The listing builds one solid part. Answer for the finished solid, in the listing's coordinates (mm). A direction names the side the tool comes from. Coordinates: 2 decimals unless noted, no trailing zeros. Order: outer loops, then holes, each group sorted by start corner. A loop starts at its lowest first (then second) coordinate and runs counter-clockwise, first axis right, second up.
```python
from build123d import *

# Parameters (mm, degrees)
F1_DEPTH = 12.7
F2_F1_R  = 5.08
F2_F2_R  = 5.08


with BuildPart() as f1:
    # F0 (on Front) → F1 (new body, symmetric)
    with BuildSketch(Plane.XZ):
        Polygon((152.4, 0), (0, 0), (0, -127), (101.6, -127), (101.6, -78.0620644748), (76.2, -78.0620644748), (76.2, -103.637776798), (50.8, -103.637776798), (50.8, -78.0620644748), (25.4, -78.0620644748), (25.4, -38.1), (127, -38.1), (127, -127), (152.4, -127), align=None)
    extrude(amount=F1_DEPTH, both=True)

    # F2: fillet of radius 5.08 on 40 edges, made by hand

    # F2_f1
    f2_f1_edges = [f1.edges().sort_by_distance(p)[0] for p in [
        (25.4, 0, -78.0620644748),
        (25.4, 0, -38.1),
        (127, 0, -38.1),
        (76.2, 0, -103.637776798),
        (50.8, 0, -103.637776798),
    ]]
    fillet(f2_f1_edges, radius=F2_F1_R)

    # F2_f2
    f2_f2_edges = [f1.edges().sort_by_distance(p)[0] for p in [
        (76.2, -12.7, 0),
        (76.2, 12.7, 0),
        (152.4, 0, 0),
        (0, 0, 0),
        (139.7, -12.7, -127),
        (152.4, 0, -127),
        (127, 0, -127),
        (139.7, 12.7, -127),
        (101.6, 0, -127),
        (50.8, -12.7, -127),
        (101.6, -12.7, -102.5310322374),
        (101.6, 12.7, -102.5310322374),
        (101.6, 0, -78.0620644748),
        (50.8, 12.7, -127),
        (0, 0, -127),
        (63.5, -12.7, -103.637776798),
        (76.2, -12.7, -88.3099206364),
        (50.8, -12.7, -88.3099206364),
        (50.8, 0, -78.0620644748),
        (50.8, 12.7, -88.3099206364),
        (63.5, 12.7, -103.637776798),
        (76.2, 0, -78.0620644748),
        (88.9, 12.7, -78.0620644748),
        (127, -12.7, -85.09),
        (127, 12.7, -85.09),
        (76.2, -12.7, -38.1),
        (25.4, -12.7, -58.0810322374),
        (40.64, -12.7, -78.0620644748),
        (0, -12.7, -63.5),
        (88.9, -12.7, -78.0620644748),
        (40.64, 12.7, -78.0620644748),
        (0, 12.7, -63.5),
        (25.4, 12.7, -58.0810322374),
        (152.4, -12.7, -63.5),
        (152.4, 12.7, -63.5),
        (26.8878975516, 12.7, -76.5741669232),
        (26.8878975516, 12.7, -39.5878975516),
        (26.8878975516, -12.7, -76.5741669232),
        (26.8878975516, -12.7, -39.5878975516),
        (125.5121024484, -12.7, -39.5878975516),
        (125.5121024484, 12.7, -39.5878975516),
        (74.7121024484, 12.7, -102.1498792464),
        (52.2878975516, 12.7, -102.1498792464),
        (52.2878975516, -12.7, -102.1498792464),
        (74.7121024484, -12.7, -102.1498792464),
    ]]
    fillet(f2_f2_edges, radius=F2_F2_R)


solid = f1.part
```
1) A cutting plane is placed at A-A, the plane z = -54. Write down the section's boundary in (x, y), plus the area to 3 significant figures.
2) A cutting plane is placed at C-C, the plane z = -91. Write down the section's boundary in (x, y).
3) A cutting plane is placed at D-D, the plane y = -0.5. Write down the section's boundary in (x, z).
4) For faces 5 (the flat face through (101.6, 0, -103)), 6 (the cylindrical face through (49.272, -11.251, -90.742)), 7 (the cylindrical face through (52.25, -0.11, -102.11)), determine the directions among +Z, -Z, +X, -X, +Y, -Y from which every point of the face is accessible in a straight line to the end or side of a thin tool.
5) The mould has two halves that part along X. Classify faces 1 (the flat face through (50, 0, -127)), 2 (the flat face through (0, 0, -63)), 3 (the flat face through (50.8, 0, -91)), 4 (the cylindrical face through (88.79, 11.25, -79.59)): released by +X, released by -X, zero draft, split by the parting line, or undercut.
6) Straight lines are drawn through the part: probe 1 along X at (y, z) = (-6.75, -96); probe 2 along X at (y, z) = (-1.25, -115); probe 3 along Z at (x, y) = (65.5, -3.5). For each, find the intervals that lie inside material, in ascending order.
7) A cutting plane is placed at B-B, the plane x = 88. Write down the section's boundary in (y, z).
8) Each of these flat-tipped pins is pushed along its axis until it touches: P1, Ø4, axis at y = 1, z = -56, coming from the -X side; P2, Ø8, axis at x = 31.5, z = -52, coming from the +Y side. Where does it stop, or does it pass through?
Working result:
1. outline: (0, -7.62) arc R5.08 ccw to (5.08, -12.7) - (20.32, -12.7) arc R5.08 ccw to (25.4, -7.62) - (25.4, 7.62) arc R5.08 ccw to (20.32, 12.7) - (5.08, 12.7) arc R5.08 ccw to (0, 7.62) - close; (127, -7.62) arc R5.08 ccw to (132.08, -12.7) - (147.32, -12.7) arc R5.08 ccw to (152.4, -7.62) - (152.4, 7.62) arc R5.08 ccw to (147.32, 12.7) - (132.08, 12.7) arc R5.08 ccw to (127, 7.62) - close
1. area: 1,250 mm2
2. outline: (0, -7.62) arc R5.08 ccw to (5.08, -12.7) - (45.72, -12.7) arc R5.08 ccw to (50.8, -7.62) - (50.8, 7.62) arc R5.08 ccw to (45.72, 12.7) - (5.08, 12.7) arc R5.08 ccw to (0, 7.62) - close; (76.2, -7.62) arc R5.08 ccw to (81.28, -12.7) - (96.52, -12.7) arc R5.08 ccw to (101.6, -7.62) - (101.6, 7.62) arc R5.08 ccw to (96.52, 12.7) - (81.28, 12.7) arc R5.08 ccw to (76.2, 7.62) - close; (127, -7.62) arc R5.08 ccw to (132.08, -12.7) - (147.32, -12.7) arc R5.08 ccw to (152.4, -7.62) - (152.4, 7.62) arc R5.08 ccw to (147.32, 12.7) - (132.08, 12.7) arc R5.08 ccw to (127, 7.62) - close
3. outline: (0, -121.92) arc R5.08 ccw to (5.08, -127) - (96.52, -127) arc R5.08 ccw to (101.6, -121.92) - (101.6, -83.14) arc R5.08 ccw to (96.52, -78.06) - (81.28, -78.06) arc R5.08 ccw to (76.2, -83.14) - (76.2, -98.56) arc R5.08 cw to (71.12, -103.64) - (55.88, -103.64) arc R5.08 cw to (50.8, -98.56) - (50.8, -83.14) arc R5.08 ccw to (45.72, -78.06) - (30.48, -78.06) arc R5.08 cw to (25.4, -72.98) - (25.4, -43.18) arc R5.08 cw to (30.48, -38.1) - (121.92, -38.1) arc R5.08 cw to (127, -43.18) - (127, -121.92) arc R5.08 ccw to (132.08, -127) - (147.32, -127) arc R5.08 ccw to (152.4, -121.92) - (152.4, -5.08) arc R5.08 ccw to (147.32, 0) - (5.08, 0) arc R5.08 ccw to (0, -5.08) - close
4. face 5: -Z, +Y, -Y
4. face 6: -Y
4. face 7: +Y, -Y
5. face 1: zero draft
5. face 2: released by -X
5. face 3: undercut
5. face 4: undercut
6. probe 1: x = 0 to 50.8, 76.2 to 101.6, 127 to 152.4
6. probe 2: x = 0 to 101.6, 127 to 152.4
6. probe 3: z = -127 to -103.64, -38.1 to 0
7. outline: (-12.7, -121.92) arc R5.08 ccw to (-7.62, -127) - (7.62, -127) arc R5.08 ccw to (12.7, -121.92) - (12.7, -83.14) arc R5.08 ccw to (7.62, -78.06) - (-7.62, -78.06) arc R5.08 ccw to (-12.7, -83.14) - close; (-12.7, -33.02) arc R5.08 ccw to (-7.62, -38.1) - (7.62, -38.1) arc R5.08 ccw to (12.7, -33.02) - (12.7, -5.08) arc R5.08 ccw to (7.62, 0) - (-7.62, 0) arc R5.08 ccw to (-12.7, -5.08) - close
8. P1: stops at x = 0
8. P2: passes through
